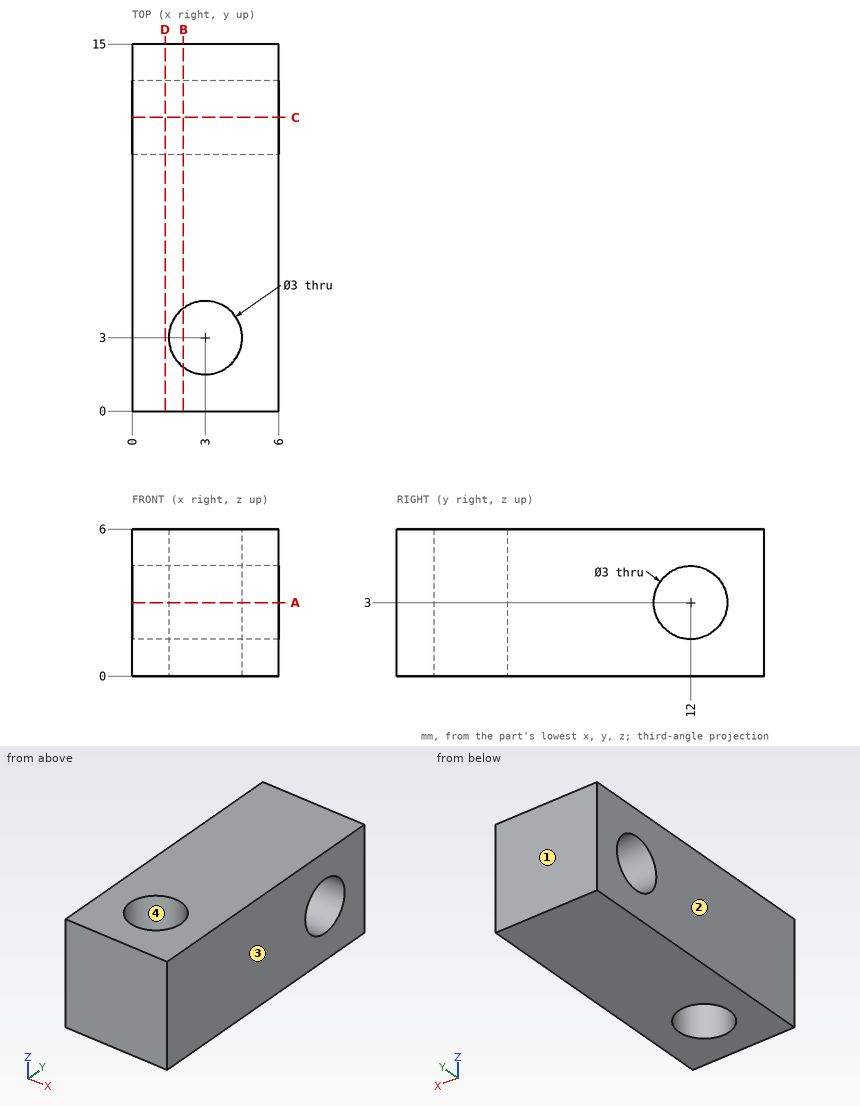
Input: dimensioned drawing with shaded views. Units: mm. Origin: part minimum x, y, z. Round coordinates to 2 decimals unless told otherwise and drop trailing zeros. Loops run counter-clockwise (first coordinate to the right, second up) from the corner with the lowest first, then second, coordinate; pieces in that order, holes last. Notation, with made-up numbers: (30, 83.25) -> (67, 83.25) arc R10 ccw to (67, 98.25) -> close; hole circle Ø7 at (-31, 51). An arc over 180 degrees is marked (long way). Answer as a JSON object with one key per item and string values. Group by question number.
Q1. Ray query, line 1 (Z direction, x = 2.2, y = 12); line 2 (Y direction, x = 3, z = 3.35); line 3 (Y direction, x = 3.2, z = 5). Return the intervals inside material, ascending. Write a range as from..to.
Q2. Mould query, pull axis X, two halves, no side actions, for the marked faces 1, 2, 3 and 4. Classes: pulls with the +X half, pulls with the -X half, needs draft (parallel to the pull), parting line crosses it, or undercut.
Q3. Contact query for a flat-ended pin moving along its axis: P1, Ø2.5, axis at y = 12, z = 3, coming from the +X side. Output: stop coordinate, or through.
Q4. Section query D-D (x = 1.35). Output: boundary loops of the cut face in (y, z), plus the area to 3 significant figures.
Q5. Section query B-B (x = 2.1). Output: boundary loops of the cut face in (y, z).
Q6. Section query C-C (y = 12). Output: boundary loops of the cut face in (x, z), plus the area to 3 significant figures.
Q7. Section query A-A (z = 3). Output: boundary loops of the cut face in (x, y), plus the area to 3 significant figures.
Completed:
{
 "1": {"line 1": "0..1.5, 4.5..6", "line 2": "0..1.5, 4.5..10.54, 13.46..15", "line 3": "0..1.51, 4.49..15"},
 "2": {"face 1": "needs draft", "face 2": "pulls with the -X half", "face 3": "pulls with the +X half", "face 4": "undercut"},
 "3": {"P1": "through"},
 "4": {"outline": "(0, 0) -> (15, 0) -> (15, 6) -> (0, 6) -> close; hole circle Ø3 at (12, 3)", "area": "82.9 mm²"},
 "5": {"outline": "(0, 0) -> (1.8, 0) -> (1.8, 6) -> (0, 6) -> close; (4.2, 0) -> (15, 0) -> (15, 6) -> (4.2, 6) -> close; hole circle Ø3 at (12, 3)"},
 "6": {"outline": "(0, 0) -> (6, 0) -> (6, 1.5) -> (0, 1.5) -> close; (0, 4.5) -> (6, 4.5) -> (6, 6) -> (0, 6) -> close", "area": "18.0 mm²"},
 "7": {"outline": "(0, 0) -> (6, 0) -> (6, 10.5) -> (0, 10.5) -> close; (0, 13.5) -> (6, 13.5) -> (6, 15) -> (0, 15) -> close; hole circle Ø3 at (3, 3)", "area": "64.9 mm²"}
}
